Check sheet for the drawn part. Datum: minimum x, y, z corner. Units: mm. A direction names the side the tool comes from. Coordinates: 2 decimals unless noted, no trailing zeros. Loops run counter-clockwise (first coordinate to the right, second up) from the corner with the lowest first, then second, coordinate; pieces in that order, holes last. Notation, with made-up numbers: M 28.5,82.25 L 61.5,82.25 A16 ccw 61.5,110.25 Z; hole C 16,10.25 d4. An arc over 180 degrees is marked long. Answer as CSV lines item,"result". Start each with the question number.
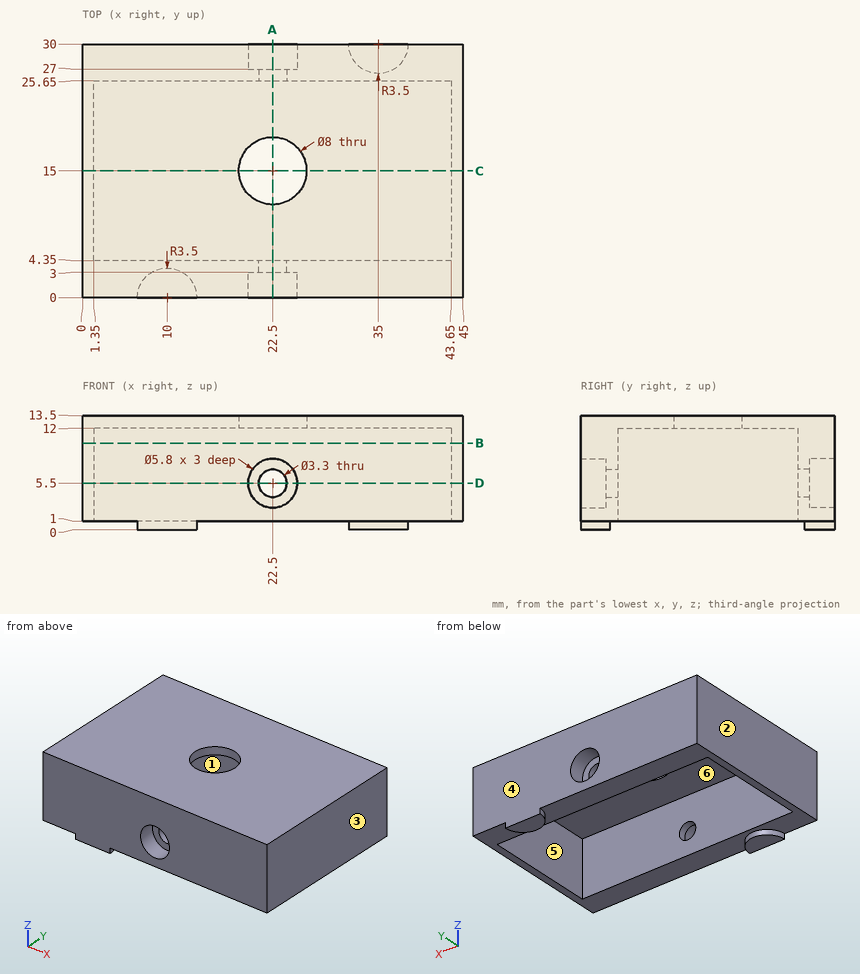
Item 1: Release check for a two-part mould opening along Y. For the marked faces 3, 4, 5 and 6 record: released by +Y, released by -Y, zero draft, split by the parting line, or undercut.
Item 2: Sectioned sample at C-C, the plane y = 15. Record the boundary of the cut face in (x, z), and give its area (3 significant figures).
Item 3: Material ranges on line 1 (Y direction, x = 33, z = 8.75); line 2 (X direction, y = 4.5, z = 7.5); line 3 (Z direction, x = 22.5, y = 3.85), recorded low to high. Write a range as from..to.
Item 4: Sectioned sample at D-D, the plane z = 5.5. Record the boundary of the cut face in (x, y), and give its area (3 significant figures).
Item 5: Go/stop test with flat-tipped pins: pin 1 (17 mm diameter, centred on x = 14.5, y = 17.5, fed in from -Z); pin 2 (2 mm diameter, centred on x = 22.5, z = 5.5, fed in from +Y); pin 3 (4.5 mm diameter, centred on x = 22.5, z = 5.5, fed in from +Y); pin 4 (1 mm diameter, centred on x = 13.5, y = 23.5, fed in from -Z). Record where each tip stops, or that it passes through.
Item 6: Sectioned sample at B-B, the plane z = 10.25. Record the boundary of the cut face in (x, y).
Item 7: Sectioned sample at A-A, the plane x = 22.5. Record the boundary of the cut face in (y, z).
Item 8: Set-up check for the marked faces 1 and 2: record each of +Z, -Z, +X, -X, +Y, -Y from which the full face is reachable in a straight line by a thin tool's end or side.
Reply:
1,face 3,"zero draft"
1,face 4,"released by +Y"
1,face 5,"undercut"
1,face 6,"undercut"
2,outline,"M 0,1 L 1.35,1 L 1.35,12 L 18.5,12 L 18.5,13.5 L 0,13.5 Z; M 26.5,12 L 43.65,12 L 43.65,1 L 45,1 L 45,13.5 L 26.5,13.5 Z"
2,area,"85.2 mm²"
3,line 1,"0..4.35, 25.65..30"
3,line 2,"0..1.35, 43.65..45"
3,line 3,"1..3.85, 7.15..13.5"
4,outline,"M 0,0 L 19.6,0 L 19.6,3 L 20.85,3 L 20.85,4.35 L 1.35,4.35 L 1.35,25.65 L 20.85,25.65 L 20.85,27 L 19.6,27 L 19.6,30 L 0,30 Z; M 24.15,3 L 25.4,3 L 25.4,0 L 45,0 L 45,30 L 25.4,30 L 25.4,27 L 24.15,27 L 24.15,25.65 L 43.65,25.65 L 43.65,4.35 L 24.15,4.35 Z"
4,area,"405 mm²"
5,pin 1,"z = 1"
5,pin 2,"through"
5,pin 3,"y = 27"
5,pin 4,"z = 12"
6,outline,"M 0,0 L 45,0 L 45,30 L 0,30 Z; hole M 1.35,4.35 L 43.65,4.35 L 43.65,25.65 L 1.35,25.65 Z"
7,outline,"M 0,1 L 4.35,1 L 4.35,3.85 L 3,3.85 L 3,2.6 L 0,2.6 Z; M 0,8.4 L 3,8.4 L 3,7.15 L 4.35,7.15 L 4.35,12 L 11,12 L 11,13.5 L 0,13.5 Z; M 19,12 L 25.65,12 L 25.65,7.15 L 27,7.15 L 27,8.4 L 30,8.4 L 30,13.5 L 19,13.5 Z; M 25.65,1 L 30,1 L 30,2.6 L 27,2.6 L 27,3.85 L 25.65,3.85 Z"
8,face 1,"-Z"
8,face 2,"+Z, -Z, -X, +Y, -Y"
